```python
from build123d import *

# Parameters (mm, degrees)
F1_DEPTH = 190.5
F2_R     = 2.6162
F3_DEPTH = 3.176
F4_R     = 2.6162
F5_DEPTH = 3.176


with BuildPart() as f1:
    # F0 (on Front) → F1 (new body)
    with BuildSketch(Plane.XZ):
        with BuildLine():
            Line((-50.8, 0), (0, 0))
            ThreePointArc((0, 0), (-0.929936, 2.245064), (-3.175, 3.175))
            Line((-3.175, 3.175), (-44.45, 3.175))
            ThreePointArc((-44.45, 3.175), (-46.695064, 4.104936), (-47.625, 6.35))
            Line((-47.625, 6.35), (-47.625, 47.625))
            ThreePointArc((-47.625, 47.625), (-48.554936, 49.870064), (-50.8, 50.8))
            Line((-50.8, 50.8), (-50.8, 0))
        make_face()
    extrude(amount=F1_DEPTH)

    # F2 (on face) → F3 (cut, through all)
    with BuildSketch(Plane.YZ.offset(-47.625)):
        with Locations((-176.2125, 14.2875)):
            Circle(F2_R)
        with Locations((-176.2125, 39.6875)):
            Circle(F2_R)
        with Locations((-150.8125, 39.6875)):
            Circle(F2_R)
        with Locations((-150.8125, 14.2875)):
            Circle(F2_R)
        with Locations((-33.6804, 42.8625)):
            Circle(F2_R)
    extrude(amount=-F3_DEPTH, mode=Mode.SUBTRACT)

    # F4 (on face) → F5 (cut, through all)
    with BuildSketch(Plane.XY.offset(3.175)):
        with Locations((-36.5125, -182.5625)):
            Circle(F4_R)
        with Locations((-36.5125, -7.9375)):
            Circle(F4_R)
        with Locations((-11.1125, -7.9375)):
            Circle(F4_R)
        with Locations((-36.5125, -33.3375)):
            Circle(F4_R)
        with Locations((-11.1125, -33.3375)):
            Circle(F4_R)
        with Locations((-36.5125, -157.1625)):
            Circle(F4_R)
        with Locations((-11.1125, -182.5625)):
            Circle(F4_R)
        with Locations((-11.1125, -157.1625)):
            Circle(F4_R)
    extrude(amount=-F5_DEPTH, mode=Mode.SUBTRACT)


solid = f1.part
```
Read the model definition and answer for the solid it produces. Units are mm, in the model's axes. Coordinates: 2 decimals unless noted, no trailing zeros. Write each loop counter-clockwise with the first axis right and the second up, starting at its lowest first coordinate (ties: lowest second). Pieces come first, ordered by that corner, then holes. Notation, with made-up numbers: (6.25, 76.5) - (54.25, 76.5) arc R12 cw to (54.25, 82.5) - close; hole circle Ø1 at (-28, -4). An arc over 180 degrees is marked (long way). Answer as a JSON object with one key per item and string values. Group by question number.
1. A cutting plane is placed at A-A (y = -166). Determine the outline of the cut face in (x, z) (3 decimals), plus the area to 3 significant figures.
2. Consider L1, parallel to Z at x = -26.5, y = -175.5 (3 decimals); L2, parallel to X at y = -39, z = 23.5 (3 decimals); L3, parallel to X at y = -82, z = 48.5. Determine where each line is inside the solid, lowest interval first. Write a range as [from, to].
3. A cutting plane is placed at C-C (z = 19). Determine the outline of the cut face in (x, y) (3 decimals), plus the area to 3 significant figures.
4. A cutting plane is placed at B-B (x = -37). Determine the outline of the cut face in (y, z) (3 decimals).
5. The mould has two halves that part along Z. Classify faces 1 (the cylindrical face through (-49.19, -36.294, 42.978)), 2 (the cylindrical face through (-36.85, -154.57, 1.61)), 3 (the flat face through (-26, -94, 0)): +Z half, -Z half, draft (parallel to the pull), parting line (faces both ways), or undercut.
6. Each of these flat-tipped pins is pushed along its axis until it touches: P1, Ø4.5, axis at x = -36.51, y = -33.34, coming from the +Z side; P2, Ø7, axis at y = -176.21, z = 14.29, coming from the +X side (3 decimals); P3, Ø1.5, axis at y = -96, z = 5.5, coming from the +X side; P4, Ø1, axis at x = -38, y = -166, coming from the +Z side (3 decimals). Where does it stop, or does it pass through?
7. A cutting plane is placed at D-D (x = -28.5). Determine the outline of the cut face in (y, z) (3 decimals).
Worked out:
{
 "1": {"outline": "(-50.8, 0) - (0, 0) arc R3.175 ccw to (-3.175, 3.175) - (-44.45, 3.175) arc R3.175 cw to (-47.625, 6.35) - (-47.625, 47.625) arc R3.175 ccw to (-50.8, 50.8) - close", "area": "310 mm²"},
 "2": {"L1": "z = [0, 3.175]", "L2": "x = [-50.8, -47.625]", "L3": "x = [-50.8, -47.75]"},
 "3": {"outline": "(-50.8, -190.5) - (-47.625, -190.5) - (-47.625, 0) - (-50.8, 0) - close", "area": "605 mm²"},
 "4": {"outline": "(-190.5, 0) - (-185.133, 0) - (-185.133, 3.175) - (-190.5, 3.175) - close; (-179.992, 0) - (-159.733, 0) - (-159.733, 3.175) - (-179.992, 3.175) - close; (-154.592, 0) - (-35.908, 0) - (-35.908, 3.175) - (-154.592, 3.175) - close; (-30.767, 0) - (-10.508, 0) - (-10.508, 3.175) - (-30.767, 3.175) - close; (-5.367, 0) - (0, 0) - (0, 3.175) - (-5.367, 3.175) - close"},
 "5": {"face 1": "undercut", "face 2": "draft", "face 3": "-Z half"},
 "6": {"P1": "passes through", "P2": "stops at x = -47.625", "P3": "stops at x = -47.19", "P4": "stops at z = 3.175"},
 "7": {"outline": "(-190.5, 0) - (0, 0) - (0, 3.175) - (-190.5, 3.175) - close"}
}
